```python
from build123d import *

# Parameters (mm, degrees)
F0_W     = 1.5875
F0_H     = 1.5875
F0_W_2   = 38.1
F1_DEPTH = 1066.8
F2_R     = 1.5875


with BuildPart() as f1:
    # F0 (on Front) → F1 (new body)
    with BuildSketch(Plane.XZ):
        with Locations((19.84375, -19.84375)):
            Rectangle(F0_W, F0_H)
        with Locations((0, -19.84375)):
            Rectangle(F0_W_2, F0_H)
        with BuildLine():
            Line((19.05, -19.05), (20.6375, -19.05))
            Line((20.6375, -19.05), (20.6375, 16.728964))
            ThreePointArc((20.6375, 16.728964), (19.70884, 19.280205), (17.357459, 20.6375))
            Line((17.357459, 20.6375), (15.980041, 20.6375))
            ThreePointArc((15.980041, 20.6375), (13.62866, 19.280205), (12.7, 16.728964))
            Line((12.7, 16.728964), (14.2875, 16.728964))
            ThreePointArc((14.2875, 16.728964), (16.66875, 19.110214), (19.05, 16.728964))
            Line((19.05, 16.728964), (19.05, -19.05))
        make_face()
        with Locations((-19.84375, -19.84375)):
            Rectangle(F0_W, F0_H)
        with BuildLine():
            Line((-20.6375, -19.05), (-19.05, -19.05))
            Line((-19.05, -19.05), (-19.05, 16.728964))
            ThreePointArc((-19.05, 16.728964), (-16.66875, 19.110214), (-14.2875, 16.728964))
            Line((-14.2875, 16.728964), (-12.7, 16.728964))
            ThreePointArc((-12.7, 16.728964), (-13.62866, 19.280205), (-15.980041, 20.6375))
            Line((-15.980041, 20.6375), (-17.357459, 20.6375))
            ThreePointArc((-17.357459, 20.6375), (-19.70884, 19.280205), (-20.6375, 16.728964))
            Line((-20.6375, 16.728964), (-20.6375, -19.05))
        make_face()
        with BuildLine():
            Line((15.980041, 20.6375), (17.357459, 20.6375))
            ThreePointArc((17.357459, 20.6375), (16.66875, 20.697714), (15.980041, 20.6375))
        make_face()
        with BuildLine():
            ThreePointArc((-15.980041, 20.6375), (-16.66875, 20.697714), (-17.357459, 20.6375))
            Line((-17.357459, 20.6375), (-15.980041, 20.6375))
        make_face()
    extrude(amount=F1_DEPTH)

    # F2
    f2_edges = [f1.edges().sort_by_distance(p)[0] for p in [
        (-19.05, -533.4, -19.05),
        (19.05, -533.4, -19.05),
        (20.6375, -533.4, -20.6375),
        (-20.6375, -533.4, -20.6375),
    ]]
    fillet(f2_edges, radius=F2_R)


solid = f1.part
```
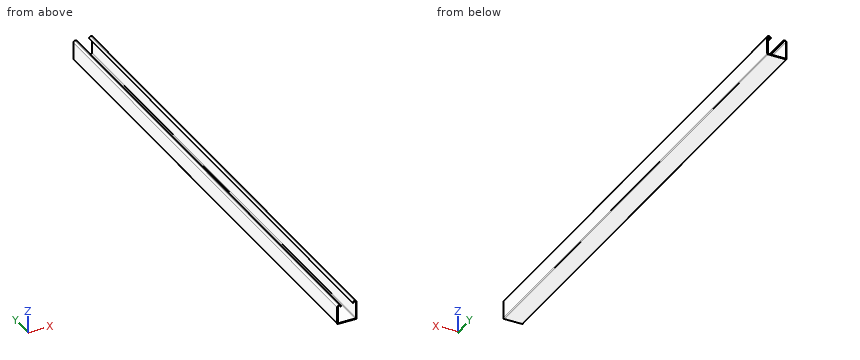
Input: part model. Units: mm. Frame: model coordinates. Give positions to 0.01 mm unless a question says otherwise; leave off trailing zeros. Order: outer loops, then holes, each group sorted by start corner. A loop starts at its lowest first (then second) coordinate and runs counter-clockwise, first axis right, second up.
1. Pin query (flat end, axial travel): pin 1 (17.5 mm diameter, centred on x = 2, y = -531.5, fed in from +Z); pin 2 (3 mm diameter, centred on x = 12, y = -853.5, fed in from +Z). Return the tip coordinate at first contact, or that it passes through.
Derived:
pin 1: stops at z = -19.05
pin 2: stops at z = 19.12
2. Section C-C on x = 1. Return the cut outline in (y, z).
Derived:
outline: (-1066.8, -20.64) - (0, -20.64) - (0, -19.05) - (-1066.8, -19.05) - close
3. Section B-B on z = -7.5. Return the cut outline in (x, y), and give its area (3 significant figures).
Derived:
outline: (-20.64, -1066.8) - (-19.05, -1066.8) - (-19.05, 0) - (-20.64, 0) - close; (19.05, -1066.8) - (20.64, -1066.8) - (20.64, 0) - (19.05, 0) - close
area: 3,390 mm2
4. Material intervals for L1, parallel to X at y = -200.5, z = -9.5; L2, parallel to X at y = -564.5, z = 18; L3, parallel to Z at x = 1, y = -175.5, sorted ascending.
Derived:
L1: x = -20.64 to -19.05, 19.05 to 20.64
L2: x = -20.43 to -18.68, -14.66 to -12.91, 12.91 to 14.66, 18.68 to 20.43
L3: z = -20.64 to -19.05
